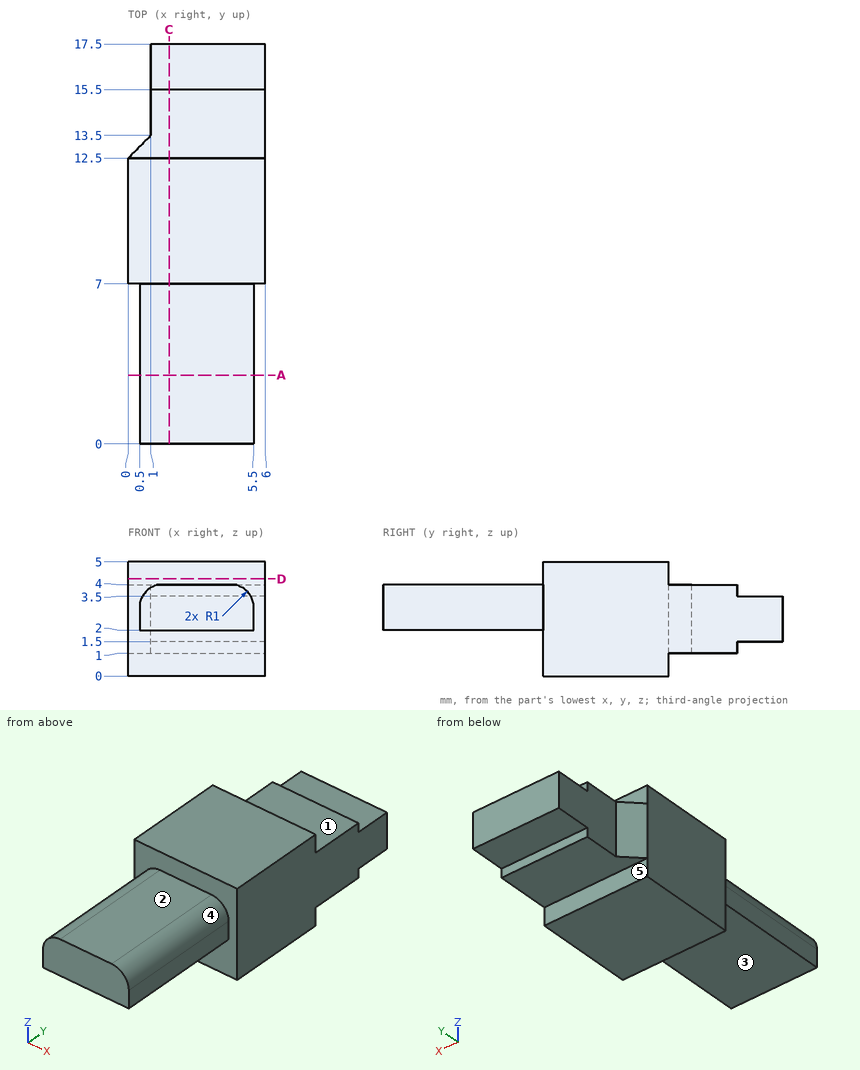
Here's the drawing with two shaded views (mm, measured from the low corner). I have some questions. A direction names the side the tool comes from. Round coordinates to 2 decimals unless told otherwise and drop trailing zeros. Write each loop counter-clockwise with the first axis right and the second up, starting at its lowest first coordinate (ties: lowest second). Pieces come first, ordered by that corner, then holes. Notation, with made-up numbers: M 18.25,31 L 38.25,31 A13 ccw 38.25,54 Z; hole C 84,9 d10. An arc over 180 degrees is marked long. Answer in a Markdown table with one row per item. Add a question column.
Q1. Will these pins go through, and if not, where does the flat tip stop? pin 1 Ø1.6 at (x, y) = (4, 16.5) entering from +Z; pin 2 Ø2.5 at (x, y) = (3, 2.5) entering from +Z; pin 3 Ø2.5 at (x, y) = (3.5, 4.5) entering from -Z.
Q2. Imagine slicing it at C-C (x = 1.8). Please give me the cut outline in (y, z), then the cut area to 3 significant figures.
Q3. Imagine slicing it at D-D (z = 4.25). Please give me the cut outline in (x, y), then the cut area to 3 significant figures.
Q4. Imagine slicing it at A-A (y = 3). Please give me the cut outline in (x, z), then the cut area to 3 significant figures.
Q5. If I drill on line 1 (Y direction, x = 3.1, z = 4.4); line 2 (Z direction, x = 4.05, y = 4.5); line 3 (Z direction, x = 2.55, y = 14.75), over which ranges is the centre line in solid material (lowest first)? Write a range as from..to.
Q6. On a 3-axis mill with a long thin cutter (end or side, diameter ignored), from which of +Z, -Z, +X, -X, +Y, -Y can I reach the whole of each face in a straight line? I mean the marked faces 1, 2, 3, 4 and 5. Say none if no direction works.
Values:
| question | item | result |
|---|---|---|
| 1 | pin 1 | z = 3.5 |
| 1 | pin 2 | z = 4 |
| 1 | pin 3 | z = 2 |
| 2 | outline | M 0,2 L 7,2 L 7,0 L 12.5,0 L 12.5,1 L 15.5,1 L 15.5,1.5 L 17.5,1.5 L 17.5,3.5 L 15.5,3.5 L 15.5,4 L 12.5,4 L 12.5,5 L 7,5 L 7,4 L 0,4 Z |
| 2 | area | 54.5 mm^2 |
| 3 | outline | M 0,7 L 6,7 L 6,12.5 L 0,12.5 Z |
| 3 | area | 33.0 mm^2 |
| 4 | outline | M 0.5,2 L 5.5,2 L 5.5,3 A1 ccw 4.5,4 L 1.5,4 A1 ccw 0.5,3 Z |
| 4 | area | 9.57 mm^2 |
| 5 | line 1 | 7..12.5 |
| 5 | line 2 | 2..4 |
| 5 | line 3 | 1..4 |
| 6 | face 1 | +Z, +X, -X, +Y |
| 6 | face 2 | +Z, +X, -X, -Y |
| 6 | face 3 | -Z, +X, -X, -Y |
| 6 | face 4 | +Z, +X, -Y |
| 6 | face 5 | -Z, +X, -X, +Y |
